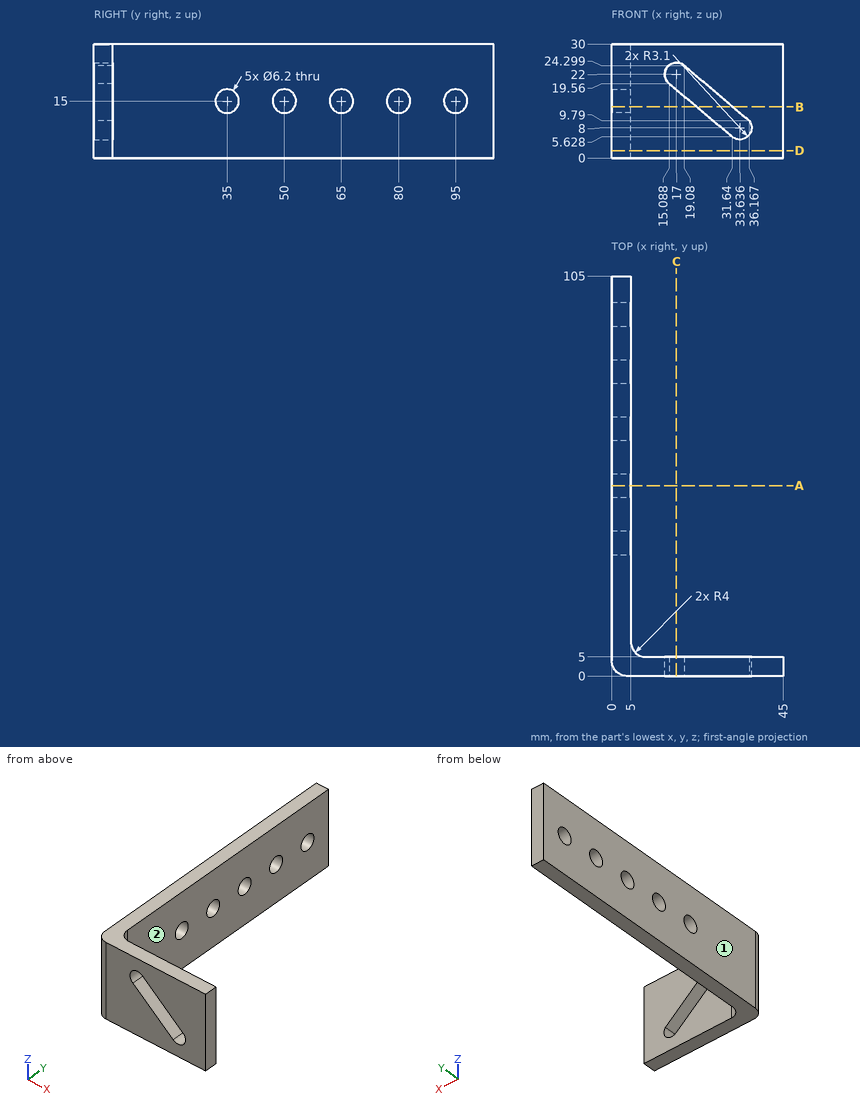
Verification items for this drawing (mm, ordinates from the low corner). A direction names the side the tool comes from. Round coordinates to 2 decimals unless told otherwise and drop trailing zeros. Write each loop counter-clockwise with the first axis right and the second up, starting at its lowest first coordinate (ties: lowest second). Pieces come first, ordered by that corner, then holes. Notation, with made-up numbers: (-16.75, -28) - (24.25, -28) arc R22 ccw to (24.25, -14) - close; hole circle Ø4 at (7, -38). An arc over 180 degrees is marked (long way). One line per item, written item: value.
1. Scan lines: L1, parallel to Y at x = 1.3, z = 15; L2, parallel to X at y = 41, z = 16. Record each from-to range of solid material in increasing order.
The answers:
L1: y = 1.05 to 31.9, 38.1 to 46.9, 53.1 to 61.9, 68.1 to 76.9, 83.1 to 91.9, 98.1 to 105
L2: x = 0 to 5
2. Cross-section at B-B on z = 13.5. Give the number of separate pieces and of enclosed holes in the cut face, and give its area (3 significant figures).
The answers:
separate pieces: 7
enclosed holes: 0
area: 542 mm^2
3. Depth check by flat-ended pin: pin 1 Ø7 at (y, z) = (95, 15) entering from +X; pin 2 Ø5 at (x, z) = (8, 27) entering from -Y; pin 3 Ø1 at (x, z) = (28, 11.5) entering from +Y; pin 4 Ø4 at (x, z) = (18.5, 26.5) entering from +Y. Enter the tip coordinate at first touch or a pass-through.
The answers:
pin 1: stops at x = 5
pin 2: stops at y = 0
pin 3: passes through
pin 4: stops at y = 5
4. Cross-section at C-C on x = 17. Record the boundary of the cut face in (y, z).
The answers:
outline: (0, 0) - (5, 0) - (5, 17.95) - (0, 17.95) - close; (0, 25.1) - (5, 25.1) - (5, 30) - (0, 30) - close
5. Set-up check for the marked faces 1 and 2: record each of +Z, -Z, +X, -X, +Y, -Y from which the full face is reachable in a straight line by a thin tool's end or side.
The answers:
face 1: +Z, -Z, -X, +Y, -Y
face 2: +Z, -Z, +X, +Y
6. Cross-section at D-D on z = 2. Record the boundary of the cut face in (x, y), and give its area (3 significant figures).
The answers:
outline: (0, 4) arc R4 ccw to (4, 0) - (45, 0) - (45, 5) - (9, 5) arc R4 cw to (5, 9) - (5, 105) - (0, 105) - close
area: 725 mm^2
7. Cross-section at A-A on y = 50. Record the boundary of the cut face in (x, z).
The answers:
outline: (0, 0) - (5, 0) - (5, 11.9) - (0, 11.9) - close; (0, 18.1) - (5, 18.1) - (5, 30) - (0, 30) - close
